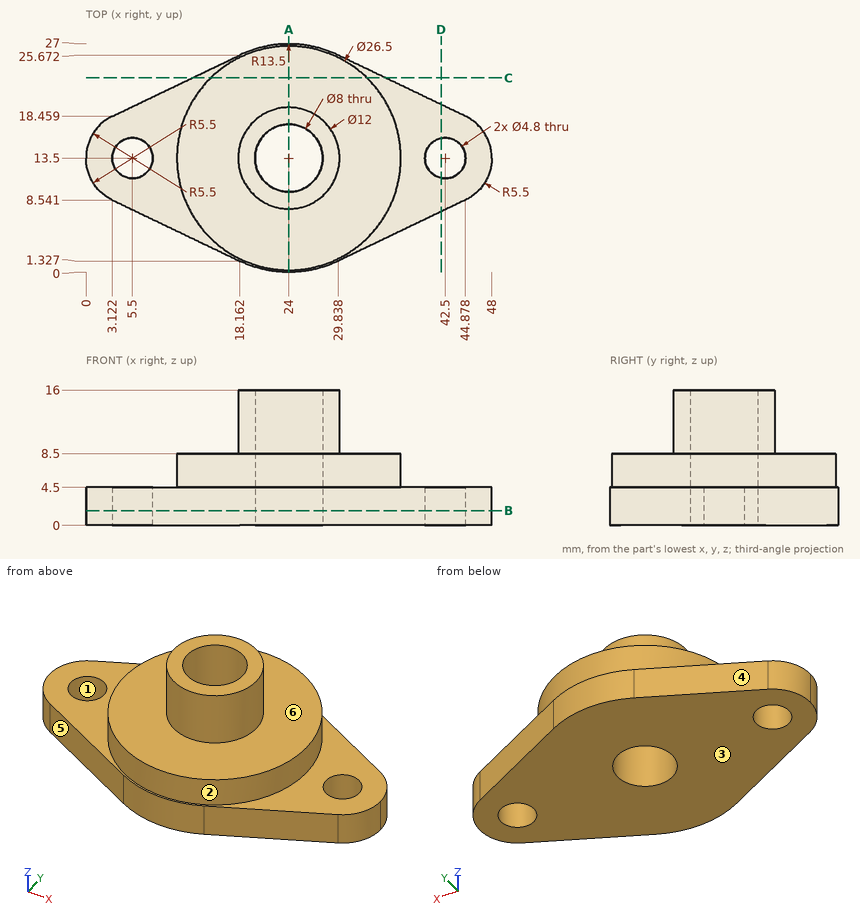
The figure shows three views and two pictorial views of one solid part (mm, origin at its lowest corner). Answer the questions. A direction names the side the tool comes from. Coordinates: 2 decimals unless noted, no trailing zeros. Loops run counter-clockwise (first coordinate to the right, second up) from the corner with the lowest first, then second, coordinate; pieces in that order, holes last. Notation, with made-up numbers: (70.25, 80) - (107.25, 80) arc R34 ccw to (107.25, 111) - close; hole circle Ø5 at (86, -22.5). An arc over 180 degrees is marked (long way). Write item = value, one per line.
1) Find the intervals of material crossed by line 1 along Y through (x, z) = (24, 12); line 2 along Z through (x, y) = (40, 19); line 3 along Z through (x, y) = (31, 9.5), in increasing order.
Responses:
line_1 = 7.5 to 9.5, 17.5 to 19.5
line_2 = 0 to 4.5
line_3 = 0 to 8.5
2) Each of these flat-tipped pins is pushed along its axis until it touches: P1, Ø1.5, axis at y = 22.5, z = 3, coming from the -X side (1 decimal); P2, Ø5, axis at y = 7.5, z = 4.5, coming from the +X side. Where does it stop, or does it pass through?
Responses:
P1 = 10
P2 = 46.74
3) Section A-A (x = 24) is taken. Determine the outline of the cut face in (y, z).
Responses:
outline = (0, 0) - (9.5, 0) - (9.5, 16) - (7.5, 16) - (7.5, 8.5) - (0.25, 8.5) - (0.25, 4.5) - (0, 4.5) - close; (17.5, 0) - (27, 0) - (27, 4.5) - (26.75, 4.5) - (26.75, 8.5) - (19.5, 8.5) - (19.5, 16) - (17.5, 16) - close
4) Section C-C (y = 23) is taken. Determine the outline of the cut face in (x, z).
Responses:
outline = (12.59, 0) - (35.41, 0) - (35.41, 4.5) - (33.24, 4.5) - (33.24, 8.5) - (14.76, 8.5) - (14.76, 4.5) - (12.59, 4.5) - close
5) Section D-D (x = 42) is taken. Determine the outline of the cut face in (y, z).
Responses:
outline = (7.16, 0) - (11.15, 0) - (11.15, 4.5) - (7.16, 4.5) - close; (15.85, 0) - (19.84, 0) - (19.84, 4.5) - (15.85, 4.5) - close
6) Determine the mould class of the marked faces 1, 2, 3 and 4 for opening direction X: pulls with the +X half, pulls with the -X half, needs draft (parallel to the pull), parting line crosses it, or undercut.
Responses:
face_1 = undercut
face_2 = parting line crosses it
face_3 = needs draft
face_4 = pulls with the -X half
7) Section B-B (z = 1.75) is taken. Determine the outline of the cut face in (x, y).
Responses:
outline = (0, 13.5) arc R5.5 ccw to (3.12, 8.54) - (18.16, 1.33) arc R13.5 ccw to (29.84, 1.33) - (44.88, 8.54) arc R5.5 ccw to (48, 13.5) arc R5.5 ccw to (44.88, 18.46) - (29.84, 25.67) arc R13.5 ccw to (18.16, 25.67) - (3.12, 18.46) arc R5.5 ccw to start; hole circle Ø4.8 at (5.5, 13.5); hole circle Ø8 at (24, 13.5); hole circle Ø4.8 at (42.5, 13.5)
8) Which of the six approach directions +Z, -Z, +X, -X, +Y, -Y give full straight-line access (tool end or side, diameter ignored) to the marked faces 5 and 6?
Responses:
face_5 = +Z, -Z, -X, -Y
face_6 = +Z
